Can you work these out from the model? Positions are in its coordinate system, mm. Face numbers are marked on the shaded views. A direction names the side the tool comes from. Coordinates: 2 decimals unless noted, no trailing zeros. Loops run counter-clockwise (first coordinate to the right, second up) from the corner with the lowest first, then second, coordinate; pieces in that order, holes last.
```python
from build123d import *

# Parameters (mm, degrees)
F1_DEPTH = 31.75
F3_D     = 9.9314


with BuildPart() as f1:
    # F0 (on Front) → F1 (new body)
    with BuildSketch(Plane.XZ):
        Polygon((0, 6.35), (0, 0), (50.8, 0), (50.8, -7.9248), (63.5, -7.9248), (63.5, 0), (120.65, 0), (120.65, 6.35), (63.5, 6.35), (63.5, 16.6624), (50.8, 16.6624), (50.8, 6.35), align=None)
    extrude(amount=F1_DEPTH)

    # F3 (through all)
    with Locations(Plane(origin=(0, 0, 0), x_dir=(1, 0, 0), z_dir=(0, 0, -1))):
        with Locations((111.125, 10.3124), (92.075, 10.3124), (28.575, 21.4376), (9.525, 21.4376)):
            Hole(F3_D / 2)


solid = f1.part
```
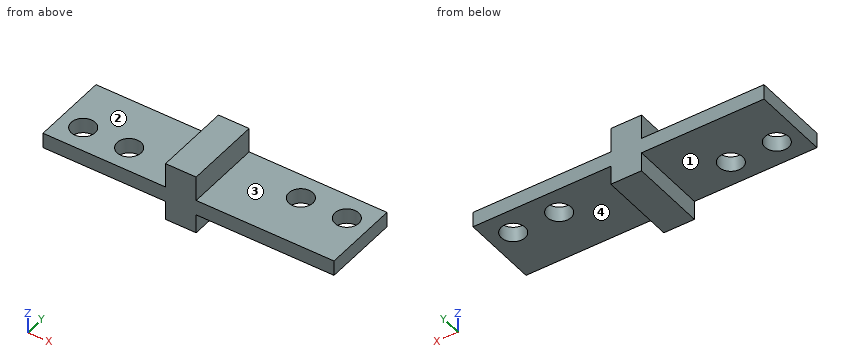
(1) I want a section at A-A on y = -20. Write out the boundary of the cut face in (x, z).
Check values:
outline: (0, 0) - (4.77, 0) - (4.77, 6.35) - (0, 6.35) - close; (14.28, 0) - (23.82, 0) - (23.82, 6.35) - (14.28, 6.35) - close; (33.33, 0) - (50.8, 0) - (50.8, -7.92) - (63.5, -7.92) - (63.5, 0) - (120.65, 0) - (120.65, 6.35) - (63.5, 6.35) - (63.5, 16.66) - (50.8, 16.66) - (50.8, 6.35) - (33.33, 6.35) - close
(2) I want a section at C-C on z = 1.25. Write out the boundary of the cut face in (x, y) (3 decimals).
Check values:
outline: (0, -31.75) - (120.65, -31.75) - (120.65, 0) - (0, 0) - close; hole circle Ø9.931 at (9.525, -21.438); hole circle Ø9.931 at (28.575, -21.438); hole circle Ø9.931 at (92.075, -10.312); hole circle Ø9.931 at (111.125, -10.312)
(3) Which directions (+Z, -Z, +X, -X, +Y, -Y) give clear straight access to the entire face, cutting with the end or side of a thin tool? Please do the marked faces 1, 2, 3 and 4.
Check values:
face 1: -Z, -X, +Y, -Y
face 2: +Z, -X, +Y, -Y
face 3: +Z, +X, +Y, -Y
face 4: -Z, +X, +Y, -Y
(4) I'm going to push flat-ended pins straight in: pin 1 (3 mm diameter, centred on y = -25, z = 12.5, fed in from -X); pin 2 (3 mm diameter, centred on x = 42.5, y = -14, fed in from -Z); pin 3 (3 mm diameter, centred on x = 47.5, z = 11, fed in from -Y); pin 4 (5 mm diameter, centred on x = 36.5, y = -3.5, fed in from +Z). Where does each tip first touch, or does it pass through?
Check values:
pin 1: stops at x = 50.8
pin 2: stops at z = 0
pin 3: passes through
pin 4: stops at z = 6.35
(5) I want a section at B-B on x = 12.5. Write out the boundary of the cut face in (y, z).
Check values:
outline: (-31.75, 0) - (-25.41, 0) - (-25.41, 6.35) - (-31.75, 6.35) - close; (-17.46, 0) - (0, 0) - (0, 6.35) - (-17.46, 6.35) - close
(6) If I drill on probe 1 along X at (y, z) = (-21, 5.75); probe 2 along X at (y, z) = (-6.5, 5.5); probe 3 along Z at (x, y) = (50.5, -26.5), over which ranges is the centre line in solid material (lowest first)?
Check values:
probe 1: x = 0 to 4.58, 14.47 to 23.63, 33.52 to 120.65
probe 2: x = 0 to 88.89, 95.26 to 107.94, 114.31 to 120.65
probe 3: z = 0 to 6.35
(7) I want a section at D-D on y = -9. Write out the boundary of the cut face in (x, z).
Check values:
outline: (0, 0) - (50.8, 0) - (50.8, -7.92) - (63.5, -7.92) - (63.5, 0) - (87.29, 0) - (87.29, 6.35) - (63.5, 6.35) - (63.5, 16.66) - (50.8, 16.66) - (50.8, 6.35) - (0, 6.35) - close; (96.86, 0) - (106.34, 0) - (106.34, 6.35) - (96.86, 6.35) - close; (115.91, 0) - (120.65, 0) - (120.65, 6.35) - (115.91, 6.35) - close
